```python
from build123d import *

# Parameters (mm, degrees)
F1_W           = 40
F1_H           = 35
F2_DEPTH       = 7
F3_R           = 10
F3_R_2         = 8
F4_DEPTH       = 3
F5_DEPTH       = 7
F6_R           = 11
F7_DEPTH       = 3
F9_D           = 3.6
F9_CBORE_D     = 6.5
F9_CBORE_DEPTH = 4
F10_D          = 2.8
F11_SIZE       = 2


with BuildPart() as f2:
    # F1 (on Top) → F2 (new body)
    with BuildSketch(Plane.XY):
        Rectangle(F1_W, F1_H)
    extrude(amount=F2_DEPTH)

    # F3 (on face) → F4 (join)
    with BuildSketch(Plane.XY.offset(7)):
        Circle(F3_R)
        Circle(F3_R_2, mode=Mode.SUBTRACT)
    extrude(amount=F4_DEPTH)

    # F5 (cut, through all): a face of the model
    f5_faces = [f2.faces().sort_by_distance(p)[0] for p in [
        (0, 0, 7),
    ]]
    extrude(f5_faces, amount=-F5_DEPTH, mode=Mode.SUBTRACT)

    # F6 (on face) → F7 (cut)
    with BuildSketch(Plane(origin=(0, 0, 0), x_dir=(1, 0, 0), z_dir=(0, 0, -1))):
        Circle(F6_R)
    extrude(amount=-F7_DEPTH, mode=Mode.SUBTRACT)

    # F9 (through all)
    with Locations(Plane.XY.offset(7)):
        with Locations((-14, 14), (14, 14), (14, -14), (-14, -14)):
            CounterBoreHole(F9_D / 2, F9_CBORE_D / 2, F9_CBORE_DEPTH)

    # F10 (through all)
    with Locations(Plane(origin=(0, 0, 0), x_dir=(1, 0, 0), z_dir=(0, 0, -1))):
        with Locations((-16.5, -9.5), (-16.5, -0.5), (16.5, -9.5), (16.5, -0.5)):
            Hole(F10_D / 2)

    # F11
    f11_edges = [f2.edges().sort_by_distance(p)[0] for p in [
        (-20, 17.5, 3.5),
        (-20, -17.5, 3.5),
        (20, 17.5, 3.5),
        (20, -17.5, 3.5),
    ]]
    chamfer(f11_edges, length=F11_SIZE)


solid = f2.part
```
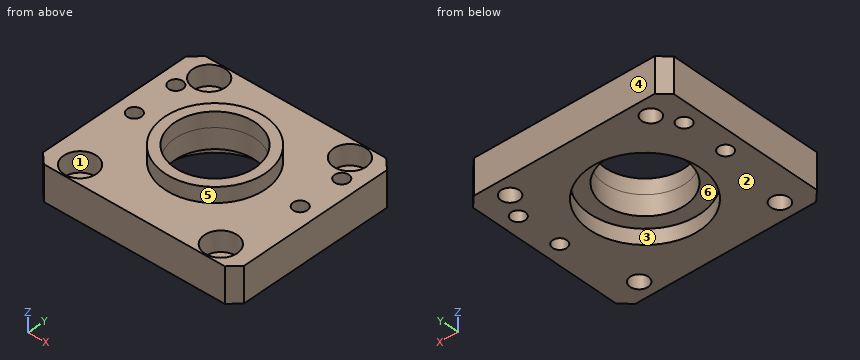
The model under review builds one solid part; all positions refer to its coordinate system, in mm. Face numbers are marked on the shaded views. A direction names the side the tool comes from. Give positions to 0.01 mm unless a question says otherwise; leave off trailing zeros. Write each loop counter-clockwise with the first axis right and the second up, starting at its lowest first coordinate (ties: lowest second). Pieces come first, ordered by that corner, then holes.
(1) To check wall thickness, follow L1, parallel to X at y = 9.5, z = 3.25; L2, parallel to Y at x = 14, z = 4.2; L3, parallel to X at y = 1.5, z = 2.5. State the ranges of each line that lie inside material, in increasing order.
(2) Tool access review of the marked faces 1, 2 and 3: name each direction out of +Z, -Z, +X, -X, +Y, -Y from which nothing blocks a thin tool from reaching the whole face with its end or side.
(3) The part is to be moulded in two halves that separate along X. For the marked faces 4, 5 and 6, say which applies: released by +X, released by -X, zero draft, split by the parting line, or undercut.
(4) Consider section D-D, the plane z = 2.25. Give the number of separate pieces and of enclosed holes in the cut face, and give its area (3 significant figures).
(5) Consider section A-A, the plane x = 14. Give the boundary of the cut face in (y, z).
(6) For P1, Ø4.5, axis at x = -14, y = -14, coming from the +Z side; P2, Ø2, axis at x = -15, y = -9.5, coming from the -Z side; P3, Ø7, axis at x = 14.5, y = 12.5, coming from the +Z side; P4, Ø11, axis at x = -5, y = -1, coming from the -Z side, all flat-tipped, find the tip position at first contact; note any pin that passes through.
(7) Consider section C-C, the plane x = 0. Give the boundary of the cut face in (y, z), and give its area (3 significant figures).
(8) Consider section B-B, the plane y = -14. Give the boundary of the cut face in (x, z).
Returned:
1. L1: x = -20 to -17.9, -15.1 to 15.1, 17.9 to 20
1. L2: y = -17.5 to -17.25, -10.75 to 10.75, 17.25 to 17.5
1. L3: x = -20 to -17.48, -15.52 to -10.9, 10.9 to 15.52, 17.48 to 20
2. face 1: +Z
2. face 2: -Z, +X, -X, +Y, -Y
2. face 3: -Z
3. face 4: zero draft
3. face 5: split by the parting line
3. face 6: undercut
4. separate pieces: 1
4. enclosed holes: 9
4. area: 947 mm2
5. outline: (-17.5, 0) - (-15.8, 0) - (-15.8, 3) - (-17.25, 3) - (-17.25, 7) - (-17.5, 7) - close; (-12.2, 0) - (12.2, 0) - (12.2, 3) - (10.75, 3) - (10.75, 7) - (-10.75, 7) - (-10.75, 3) - (-12.2, 3) - close; (15.8, 0) - (17.5, 0) - (17.5, 7) - (17.25, 7) - (17.25, 3) - (15.8, 3) - close
6. P1: stops at z = 3
6. P2: stops at z = 0
6. P3: stops at z = 7
6. P4: stops at z = 3
7. outline: (-17.5, 0) - (-11, 0) - (-11, 3) - (-8, 3) - (-8, 10) - (-10, 10) - (-10, 7) - (-17.5, 7) - close; (8, 3) - (11, 3) - (11, 0) - (17.5, 0) - (17.5, 7) - (10, 7) - (10, 10) - (8, 10) - close
7. area: 127 mm2
8. outline: (-20, 0) - (-15.8, 0) - (-15.8, 3) - (-17.25, 3) - (-17.25, 7) - (-20, 7) - close; (-12.2, 0) - (12.2, 0) - (12.2, 3) - (10.75, 3) - (10.75, 7) - (-10.75, 7) - (-10.75, 3) - (-12.2, 3) - close; (15.8, 0) - (20, 0) - (20, 7) - (17.25, 7) - (17.25, 3) - (15.8, 3) - close
